```python
from build123d import *

# Parameters (mm, degrees)
EXTRUDE_1_DEPTH     = 2.6
FILLET_1_R          = 2
SKETCH_2_W          = 2.6
SKETCH_2_H          = 2.6
SKETCH_2_R          = 0.6
EXTRUDE_2_DEPTH     = 1.5
SKETCH_3_W          = 2.6
SKETCH_3_H          = 0.5
CUT_EXTRUDE_1_DEPTH = 12.340634903


with BuildPart() as part:
    # 草图1 → 凸台-拉伸1 (new body)
    with BuildSketch(Plane.XY):
        Polygon((6.6, 6.1), (-6.6, 6.1), (-6.6, -6.1), (-5, -6.1), (-5, 5.1), (5, 5.1), (5, -6.1), (6.6, -6.1), align=None)
    extrude(amount=EXTRUDE_1_DEPTH)

    # 圆角1
    fillet_1_edges = [part.edges().sort_by_distance(p)[0] for p in [
        (5, 5.1, 1.3),
        (-5, 5.1, 1.3),
        (-6.6, 6.1, 1.3),
        (6.6, 6.1, 1.3),
    ]]
    fillet(fillet_1_edges, radius=FILLET_1_R)

    # 草图2 → 凸台-拉伸2 (add)
    # profile 1 of 2: a face of its own
    with BuildSketch(Plane.XZ.offset(6.1)):
        with Locations((-7.9, 1.3)):
            Rectangle(SKETCH_2_W, SKETCH_2_H)
        with Locations(Location((-7.9, 1.3, 0), (0, 0, 270))):
            Circle(SKETCH_2_R, mode=Mode.SUBTRACT)
    # profile 2 of 2: a face of its own
    with BuildSketch(Plane.XZ.offset(6.1)):
        with Locations((7.9, 1.3)):
            Rectangle(SKETCH_2_W, SKETCH_2_H)
        with Locations(Location((7.9, 1.3, 0), (0, 0, 270))):
            Circle(SKETCH_2_R, mode=Mode.SUBTRACT)
    extrude(amount=-EXTRUDE_2_DEPTH)

    # 草图3 → 切除-拉伸1 (cut, through all)
    with BuildSketch(Plane(origin=(0, 0, 0), x_dir=(-1, 0, 0), z_dir=(0, 0, -1))):
        with Locations((7.9, -4.85)):
            Rectangle(SKETCH_3_W, SKETCH_3_H)
    extrude(amount=-CUT_EXTRUDE_1_DEPTH, mode=Mode.SUBTRACT)


solid = part.part
```
Could you check a few things on this model? Use its own coordinates, in mm. A direction names the side the tool comes from. Round coordinates to 2 decimals unless told otherwise and drop trailing zeros. Loops run counter-clockwise (first coordinate to the right, second up) from the corner with the lowest first, then second, coordinate; pieces in that order, holes last.
Q1. For P1, Ø1.5, axis at y = 3.5, z = 2.5, coming from the -X side; P2, Ø1.3, axis at x = 1, z = 0.5, coming from the -Y side; P3, Ø1.4, axis at x = 7.9, z = 1.3, coming from the +Y side, each with a flat end and sliding along its axis, tell me the tip position at first contact or that it passes through.
Q2. Please list where these lines run through material, in increasing order: L1, parallel to X at y = -5.5, z = 1.3; L2, parallel to X at y = -2.75, z = 0.4; L3, parallel to X at y = 4, z = 1.7.
Q3. I want a section at C-C (z = 1.3). Write out the boundary of the cut face in (x, y), and give its area (3 significant figures).
Q4. I want a section at B-B (x = 7.9). Write out the boundary of the cut face in (y, z).
Q5. On a 3-axis mill with a long thin cutter (end or side, diameter ignored), from which of +Z, -Z, +X, -X, +Y, -Y can I reach the whole of each face in a straight line? I mean faces 1 (the flat face through (0, 5.4, 0)), 2 (the flat face through (-7, -5.1, 1)), 3 (the cylindrical face through (-4.43, 4.5, 1.32)). Say none if no direction works.
Q6. I want a section at D-D (z = 2.2). Write out the boundary of the cut face in (x, y).
Q7. Thinking about a two-plate mould opening in X: for faces 4 (the cylindrical face through (-8.265, -5.607, 1.776)), 5 (the cylindrical face through (-6, 5.53, 1.32)), 6 (the flat face through (6.6, 0, 1)), 7 (the flat face through (0, 5.4, 2.6)), which applies, pulls with the +X half, pulls with the -X half, needs draft (parallel to the pull), parting line crosses it, or undercut?
Q8. I want a section at A-A (y = -2.5). Write out the boundary of the cut face in (x, z).
Answer below:
1. P1: stops at x = -6.6
1. P2: stops at y = 5.1
1. P3: stops at y = -4.6
2. L1: x = -9.2 to -8.5, -7.3 to -5, 5 to 7.3, 8.5 to 9.2
2. L2: x = -6.6 to -5, 5 to 6.6
2. L3: x = -6.6 to -4.79, 4.79 to 6.6
3. outline: (-9.2, -6.1) - (-8.5, -6.1) - (-8.5, -5.1) - (-9.2, -5.1) - close; (-7.3, -6.1) - (-5, -6.1) - (-5, 3.1) arc R2 cw to (-3, 5.1) - (3, 5.1) arc R2 cw to (5, 3.1) - (5, -6.1) - (7.3, -6.1) - (7.3, -4.6) - (6.6, -4.6) - (6.6, 4.1) arc R2 ccw to (4.6, 6.1) - (-4.6, 6.1) arc R2 ccw to (-6.6, 4.1) - (-6.6, -5.1) - (-7.3, -5.1) - close; (8.5, -6.1) - (9.2, -6.1) - (9.2, -4.6) - (8.5, -4.6) - close
3. area: 52.5 mm2
4. outline: (-6.1, 0) - (-4.6, 0) - (-4.6, 0.7) - (-6.1, 0.7) - close; (-6.1, 1.9) - (-4.6, 1.9) - (-4.6, 2.6) - (-6.1, 2.6) - close
5. face 1: -Z, +X, -X, +Y, -Y
5. face 2: +Z, -Z, -X, +Y
5. face 3: +Z, -Z, -Y
6. outline: (-9.2, -6.1) - (-5, -6.1) - (-5, 3.1) arc R2 cw to (-3, 5.1) - (3, 5.1) arc R2 cw to (5, 3.1) - (5, -6.1) - (9.2, -6.1) - (9.2, -4.6) - (6.6, -4.6) - (6.6, 4.1) arc R2 ccw to (4.6, 6.1) - (-4.6, 6.1) arc R2 ccw to (-6.6, 4.1) - (-6.6, -5.1) - (-9.2, -5.1) - close
7. face 4: undercut
7. face 5: pulls with the -X half
7. face 6: pulls with the +X half
7. face 7: needs draft
8. outline: (-6.6, 0) - (-5, 0) - (-5, 2.6) - (-6.6, 2.6) - close; (5, 0) - (6.6, 0) - (6.6, 2.6) - (5, 2.6) - close
